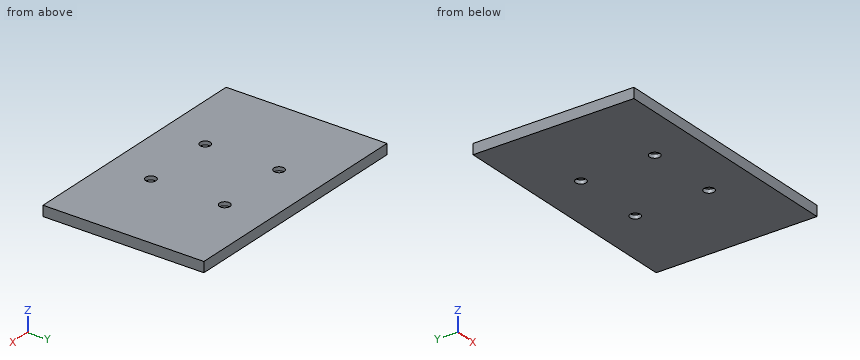
```python
from build123d import *

# Parameters (mm, degrees)
SKETCH1_W           = 168.5
SKETCH1_H           = 109
BOSS_EXTRUDE1_DEPTH = 7
SKETCH2_R           = 3.493429644
CUT_EXTRUDE1_DEPTH  = 2.5


with BuildPart() as part:
    # Sketch1 → Boss-Extrude1 (new body)
    with BuildSketch(Plane(origin=(0, 0, 0), x_dir=(-1, 0, 0), z_dir=(0, 0, 1))):
        with Locations((0, -15.7805)):
            Rectangle(SKETCH1_W, SKETCH1_H)
    extrude(amount=BOSS_EXTRUDE1_DEPTH)

    # Sketch2 → Cut-Extrude1 (cut)
    with BuildSketch(Plane.XY.offset(7)):
        with Locations((25, 40.7805)):
            Circle(SKETCH2_R)
        with Locations((-25, 40.7805)):
            Circle(SKETCH2_R)
        with Locations((-25, -9.2195)):
            Circle(SKETCH2_R)
        with Locations((25, -9.2195)):
            Circle(SKETCH2_R)
    cut_extrude1 = extrude(amount=-CUT_EXTRUDE1_DEPTH, mode=Mode.SUBTRACT)

    # Mirror1: Cut-Extrude1 across plane
    add(cut_extrude1.mirror(Plane.XY.offset(3.5)), mode=Mode.SUBTRACT)


solid = part.part
```
Read the model definition and answer for the solid it produces. Units are mm, in the model's axes. Coordinates: 2 decimals unless noted, no trailing zeros. Order: outer loops, then holes, each group sorted by start corner. A loop starts at its lowest first (then second) coordinate and runs counter-clockwise, first axis right, second up. Notation, with made-up numbers: (85, -14.75) - (112, -14.75) arc R31 ccw to (112, 17.25) - close; hole circle Ø7 at (44.5, -24). An arc over 180 degrees is marked (long way). Answer as a JSON object with one key per item and string values. Group by question number.
Item 1: Section A-A (x = -25) is taken. Give the vertices of the cut face in (y, z), plus the area to 3 significant figures.
Item 2: Consider probe 1 along Y at (x, z) = (-25, 6.25); probe 2 along X at (y, z) = (-6, 5). Determine where each line is inside the solid, lowest interval first. Write a range as from..to.
Item 3: Flat-ended cylindrical pins translate along their axes: P1, Ø2, axis at x = -25.5, y = -8, coming from the -Z side; P2, Ø3.5, axis at x = -24, y = 40.5, coming from the +Z side. Find the tip coordinate at first contact, or state that the pin passes through.
Results are:
{
 "1": {"outline": "(-38.72, 0) - (-12.71, 0) - (-12.71, 2.5) - (-5.73, 2.5) - (-5.73, 0) - (37.29, 0) - (37.29, 2.5) - (44.27, 2.5) - (44.27, 0) - (70.28, 0) - (70.28, 7) - (44.27, 7) - (44.27, 4.5) - (37.29, 4.5) - (37.29, 7) - (-5.73, 7) - (-5.73, 4.5) - (-12.71, 4.5) - (-12.71, 7) - (-38.72, 7) - close", "area": "693 mm^2"},
 "2": {"probe 1": "y = -38.72..-12.71, -5.73..37.29, 44.27..70.28", "probe 2": "x = -84.25..-26.36, -23.64..23.64, 26.36..84.25"},
 "3": {"P1": "stops at z = 2.5", "P2": "stops at z = 4.5"}
}
